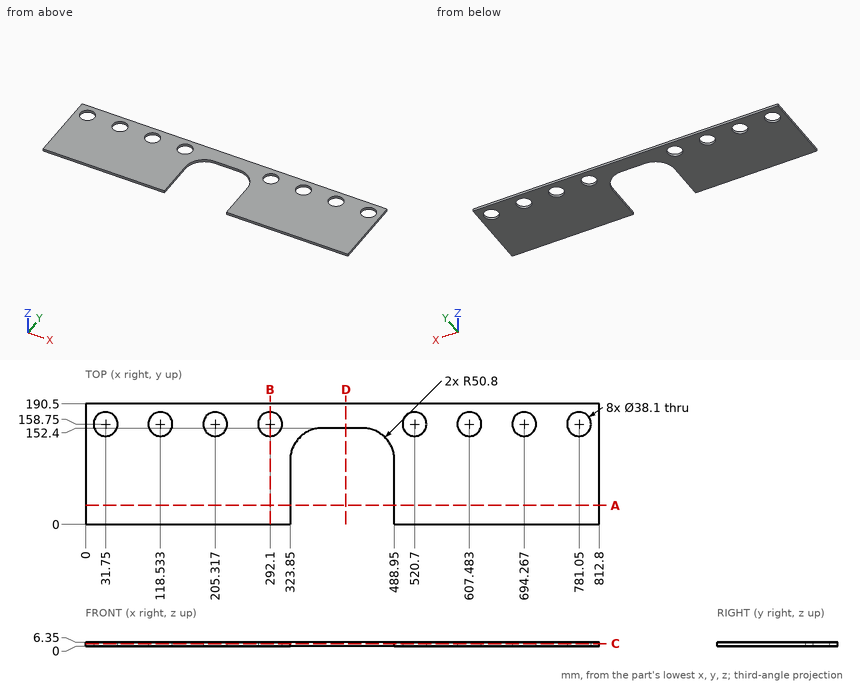
Input: dimensioned drawing with shaded views. Units: mm. Origin: part minimum x, y, z. Coordinates: 2 decimals unless noted, no trailing zeros. Loops run counter-clockwise (first coordinate to the right, second up) from the corner with the lowest first, then second, coordinate; pieces in that order, holes last. Notation, with made-up numbers: (-35.5, 22.5) -> (-6.5, 22.5) arc R29 ccw to (-6.5, 61.5) -> close; hole circle Ø4 at (46, 87.5). An arc over 180 degrees is marked (long way). One line per item, written item: value. Start each with the question number.
Q1. Section query A-A, the plane y = 30. Return the cut outline in (x, z).
Q2. Section query B-B, the plane x = 292.1. Return the cut outline in (y, z), and give its area (3 significant figures).
Q3. Section query D-D, the plane x = 412. Return the cut outline in (y, z), and give its area (3 significant figures).
Q4. Section query C-C, the plane z = 4.25. Give the number of separate pieces and of enclosed holes in the cut face, and give its area (3 significant figures).
Q5. Line query: line 1 along X through (y, z) = (89.5, 6); line 2 along Y through (x, z) = (31.75, 4); line 3 along Y through (x, z) = (409, 6). Output: solid intervals per line, ascending.
Results:
1. outline: (0, 0) -> (323.85, 0) -> (323.85, 6.35) -> (0, 6.35) -> close; (488.95, 0) -> (812.8, 0) -> (812.8, 6.35) -> (488.95, 6.35) -> close
2. outline: (0, 0) -> (139.7, 0) -> (139.7, 6.35) -> (0, 6.35) -> close; (177.8, 0) -> (190.5, 0) -> (190.5, 6.35) -> (177.8, 6.35) -> close
2. area: 968 mm^2
3. outline: (152.4, 0) -> (190.5, 0) -> (190.5, 6.35) -> (152.4, 6.35) -> close
3. area: 242 mm^2
4. separate pieces: 1
4. enclosed holes: 8
4. area: 122,000 mm^2
5. line 1: 0 to 323.85, 488.95 to 812.8
5. line 2: 0 to 139.7, 177.8 to 190.5
5. line 3: 152.4 to 190.5
